Verification items for the finished model (mm, model axes). A direction names the side the tool comes from. Round coordinates to 2 decimals unless told otherwise and drop trailing zeros. Loops run counter-clockwise (first coordinate to the right, second up) from the corner with the lowest first, then second, coordinate; pieces in that order, holes last. Notation, with made-up numbers: M 45.5,-27 L 86.5,-27 A24 cw 86.5,2 Z; hole C 34.5,70 d11. An arc over 180 degrees is marked long. One line per item, written item: value.
Autodesk Fusion 360 part; units mm, degrees
sketch "草图1" plane through (0, 0, 0) normal (0, 0, 1) x (1, 0, 0)
  circle A0 centre (0, 22) radius 4
  circle A1 centre (0, 22) radius 8
  line L0 (-8, 22) -> (-8, 0)
  line L1 (-8, 0) -> (8, 0)
  line L2 (8, 0) -> (8, 22)
  line L3 (0, 108.3744) -> (0, -35) construction
  dimension "d1" = 8
  dimension "d2" = 16
  dimension "d3" = 22
extrude "拉伸1" add sketch "草图1" along normal mid plane 16
sketch "草图2" plane through (8, 0, 0) normal (1, 0, 0) x (0, 1, 0)
  line L0 (22, -8) -> (22, 8)
  line L1 (22, 8) -> (0, 8)
  line L2 (0, 8) -> (0, -8)
  line L3 (0, -8) -> (22, -8)
  circle A0 centre (8, 0) radius 8
  circle A1 centre (8, 0) radius 4
  line L4 (8, 8) -> (22, 8)
  line L5 (22, 8) -> (22, -8)
  line L6 (8, -8) -> (22, -8)
  line L7 (-6, 0) -> (34.5187, 0) construction
  dimension "d6" = 16
  dimension "d7" = 8
  dimension "d8" = 14
extrude "拉伸2" cut sketch "草图2" against normal blind 52 contours L2 L3 A0 | L1 L2 A0 | A1
sketch "草图3" plane through (8, 0, 0) normal (1, 0, 0) x (0, 1, 0)
  circle A0 centre (8, 0) radius 4
  arc A1 (8, 8) -> (8, -8) centre (8, 0) ccw
  line L0 (8, -8) -> (22, -8)
  line L1 (22, -8) -> (22, 8)
  line L2 (22, 8) -> (8, 8)
  line L3 (17, 3) -> (30, 3)
  line L4 (30, 3) -> (30, -3)
  line L5 (30, -3) -> (17, -3)
  line L6 (17, -3) -> (17, 3)
  line L7 (-4, 0) -> (38.4958, 0) construction
  line L8 (30, 8) -> (30, -8) construction
  dimension "d11" = 6
  dimension "d12" = 13
extrude "拉伸3" cut sketch "草图3" against normal blind 21 contours L1 L3 L4 L5 | L1 L3 L5 L6
sketch "草图4" plane through (0, 0, 8) normal (0, 0, 1) x (-1, 0, 0)
  line L0 (8, -8) -> (-8, -8)
  line L1 (-8, -8) -> (-8, -22)
  arc A0 (-8, -22) -> (8, -22) centre (0, -22) ccw
  line L2 (8, -22) -> (8, -8)
  circle A1 centre (0, -22) radius 4
  line L3 (-3, 0) -> (3, 0)
  line L4 (3, 0) -> (3, -13)
  line L5 (3, -13) -> (-3, -13)
  line L6 (-3, -13) -> (-3, 0)
  line L7 (0, 5) -> (0, -37) construction
  line L8 (-8, 0) -> (8, 0) construction
  dimension "d15" = 6
  dimension "d16" = 13
extrude "拉伸4" cut sketch "草图4" against normal blind 68 contours L0 L4 L5 L6 | L0 L3 L4 L6
(1) Mould release check, pull along Y, two halves, no side actions. Record for faces 1 (the face through (5.5, 4.8, -2.4)), 2 (the face through (0.1, 26.5, -3)), 3 (the face through (0, 30, 5)), 4 (the face through (-0.521, 18.034, -5.535)): +Y half, -Y half, draft (parallel to the pull), parting line (faces both ways), or undercut.
Completed:
face 1: undercut
face 2: draft
face 3: +Y half
face 4: undercut
(2) Sectioned sample at B-B on z = 0. Enter the section's corners in (x, y).
Completed:
outline: M -8,0 L -3,0 L -3,4 L -8,4 Z; M -8,12 L -3,12 L -3,13 L 3,13 L 3,12 L 8,12 L 8,17 L -8,17 Z; M 3,0 L 8,0 L 8,4 L 3,4 Z
(3) Depth check by flat-ended pin: pin 1 Ø1 at (x, z) = (4.5, -4.5) entering from -Y; pin 2 Ø3 at (x, z) = (2.5, -4.5) entering from +Y; pin 3 Ø3 at (x, z) = (0, -4.5) entering from -Y; pin 4 Ø5 at (x, y) = (-1, 20) entering from +Z. Enter the tip coordinate at first touch or a pass-through.
Completed:
pin 1: stops at y = 1.07
pin 2: stops at y = 29.94
pin 3: stops at y = 13
pin 4: stops at z = 8
(4) Tool access check on faces 5 (the face through (3, 3.7, 0.1)), 6 (the face through (0.1, 26.3, 3)), 7 (the face through (0, 30, -6)). Record the directions out of +Z, -Z, +X, -X, +Y, -Y that give a thin tool (end or side, any length) a straight path to the whole face; none if there is none.
Completed:
face 5: +Z, -Z, -Y
face 6: +X, -X, +Y
face 7: +Z, -Z, +Y
(5) Sectioned sample at C-C on x = 0. Enter the section's corners in (y, z).
Completed:
outline: M 13,-8 L 18,-8 L 18,-3 L 17,-3 L 17,3 L 18,3 L 18,8 L 13,8 Z; M 26,-8 L 30,-8 L 30,-3 L 26,-3 Z; M 26,3 L 30,3 L 30,8 L 26,8 Z
(6) Thickness scan on L1, parallel to X at y = 7.5, z = -4.25; L2, parallel to X at y = 22, z = -6. Record the ranges inside material, lowest first. Write a range as from..to.
Completed:
L1: x = -8..-3, 3..8
L2: x = -8..-4, 4..8
(7) Sectioned sample at D-D on z = -5.5. Enter the section's corners in (x, y), and give its area (3 significant figures).
Completed:
outline: M -8,2.19 L -3,2.19 L -3,13 L 3,13 L 3,2.19 L 8,2.19 L 8,22 A8 ccw -8,22 Z; hole C 0,22 d8
area: 302 mm^2
(8) Sectioned sample at A-A on y = 7. Enter the section's corners in (x, z), and give its area (3 significant figures).
Completed:
outline: M -8,-7.94 L -3,-7.94 L -3,-3.87 L -8,-3.87 Z; M -8,3.87 L -3,3.87 L -3,7.94 L -8,7.94 Z; M 3,-7.94 L 8,-7.94 L 8,-3.87 L 3,-3.87 Z; M 3,3.87 L 8,3.87 L 8,7.94 L 3,7.94 Z
area: 81.3 mm^2
